The listing builds one solid part. Answer for the finished solid, in the listing's coordinates (mm). A direction names the side the tool comes from. Give positions to 0.01 mm unless a question says otherwise; leave off trailing zeros. Write each loop counter-clockwise with the first axis right and the second up, starting at its lowest first coordinate (ties: lowest second). Pieces come first, ordered by that corner, then holes.
Autodesk Inventor part; units mm, degrees
ref_plane "YZ Plane" through (0, 0, 0) normal (1, 0, 0) x (0, 1, 0)
ref_plane "XZ Plane" through (0, 0, 0) normal (0, 1, 0) x (-1, 0, 0)
ref_plane "XY Plane" through (0, 0, 0) normal (0, 0, 1) x (1, 0, 0)
sketch "Sketch1" plane through (0, 0, 0) normal (0, 1, 0) x (-1, 0, 0)
  line L0 (0, 0) -> (12, 0)
  line L1 (12, 0) -> (12, 10)
  line L2 (12, 10) -> (0, 10)
  line L3 (0, 10) -> (0, 0)
  line L4 (0, 0) -> (10, 0)
  line L5 (10, 0) -> (10, 2)
  line L6 (10, 2) -> (0, 2)
  line L7 (0, 2) -> (0, 0)
  dimension "d0" = 12
  dimension "d1" = 10
  dimension "d2" = 10
  dimension "d3" = 2
extrude "Extrusion1" add sketch "Sketch1" along normal blind 2 contours L5 L6 L3 L2 L1 L0
properties part number "Bocks"
Item 1: A cutting plane is placed at C-C, the plane x = -0.75. Give the vertices of the cut face in (y, z), plus the area to 3 significant figures.
Conclusion:
outline: (0, 2) - (2, 2) - (2, 10) - (0, 10) - close
area: 16.0 mm2
Item 2: Which of the six approach directions +Z, -Z, +X, -X, +Y, -Y give full straight-line access (tool end or side, diameter ignored) to faces 1 (the face through (-5, 1, 2)), 2 (the face through (-6, 0, 6))?
Conclusion:
face 1: -Z, +X, +Y, -Y
face 2: +Z, -Z, +X, -X, -Y
Item 3: Each of these flat-tipped pins is pushed along its axis until it touches: P1, Ø0.6, axis at y = 0.5, z = 1.5, coming from the +X side; P2, Ø1, axis at x = -8, y = 1, coming from the -Z side. Where does it stop, or does it pass through?
Conclusion:
P1: stops at x = -10
P2: stops at z = 2
Item 4: Consider probe 1 along Z at (x, y) = (-0.75, 1.5); probe 2 along X at (y, z) = (0.2, 1). Determine where each line is inside the solid, lowest interval first.
Conclusion:
probe 1: z = 2 to 10
probe 2: x = -12 to -10
Item 5: A cutting plane is placed at B-B, the plane z = 1.75. Give the vertices of the cut face in (x, y).
Conclusion:
outline: (-12, 0) - (-10, 0) - (-10, 2) - (-12, 2) - close
Item 6: A cutting plane is placed at A-A, the plane y = 0.3. Give the vertices of the cut face in (x, z), plus the area to 3 significant figures.
Conclusion:
outline: (-12, 0) - (-10, 0) - (-10, 2) - (0, 2) - (0, 10) - (-12, 10) - close
area: 100 mm2
